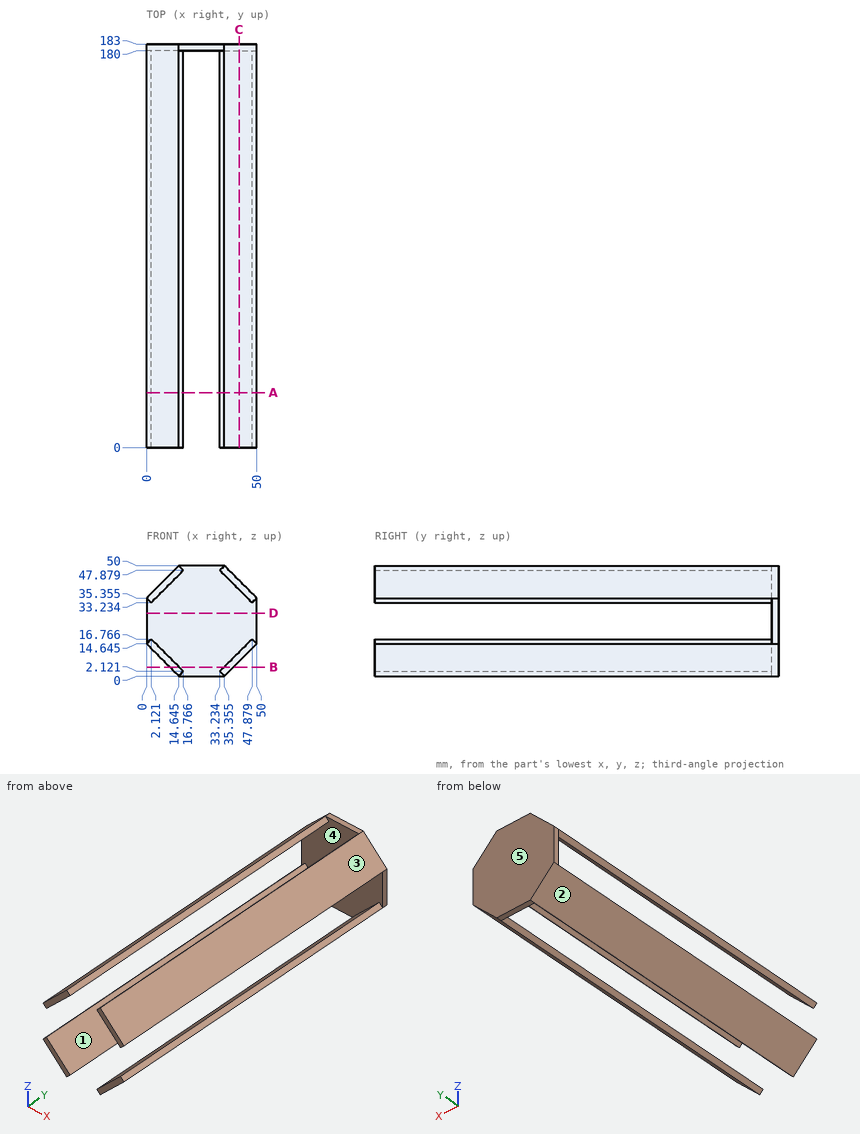
Print and shaded views of the part. All mm, measured from the part's lowest x, y and z. A direction names the side the tool comes from. Coordinates: 2 decimals unless noted, no trailing zeros. Order: outer loops, then holes, each group sorted by start corner. A loop starts at its lowest first (then second) coordinate and runs counter-clockwise, first axis right, second up. Notation, with made-up numbers: (77, -13.5) - (81, -13.5) arc R8 ccw to (81, 1.5) - close; hole circle Ø1 at (51.25, 14). An arc over 180 degrees is marked (long way). Put each result on its own line as item: value.
1. Saw through at D-D (z = 28.5). Write the cut outline in (x, y), and give its area (3 significant figures).
Answer sheet:
outline: (0, 180) - (50, 180) - (50, 183) - (0, 183) - close
area: 150 mm^2
2. Tool access for the marked faces 4 and 5: list every direction of +Z, -Z, +X, -X, +Y, -Y with a clear straight run to the whole face (end or side of a thin tool).
Answer sheet:
face 4: -Y
face 5: +Z, -Z, +X, -X, +Y
3. Drop flat-ended pins along their axis: P1, Ø6, axis at x = 27.5, z = 22.5, coming from the -Y side; P2, Ø1.5, axis at y = 77.5, z = 40, coming from the -X side (1 decimal); P3, Ø10, axis at x = 30, y = 26.5, coming from the -Z side (1 decimal). Give the stop position or say it passes through.
Answer sheet:
P1: stops at y = 180
P2: stops at x = 3.9
P3: stops at z = 0.4
4. Pull direction Z, two halves, no side cores. Call the marked faces 1, 2 and 3: pulls with the +Z half, pulls with the -Z half, needs draft (parallel to the pull), parting line crosses it, or undercut.
Answer sheet:
face 1: undercut
face 2: pulls with the -Z half
face 3: pulls with the +Z half
5. Probe line 1 along Y through (x, z) = (36, 19); line 2 along X through (y, z) = (116, 42.5) (1 decimal); line 3 along Z through (x, y) = (38, 100) (1 decimal). List the from-to ranges inside material, lowest first. Write a range as [from, to].
Answer sheet:
line 1: y = [180, 183]
line 2: x = [7.1, 11.4], [38.6, 42.9]
line 3: z = [2.6, 6.9], [43.1, 47.4]
6. Saw through at C-C (x = 42). Write the cut outline in (y, z) (1 decimal), and give its area (3 significant figures).
Answer sheet:
outline: (0, 6.6) - (183, 6.6) - (183, 43.4) - (0, 43.4) - (0, 39.1) - (180, 39.1) - (180, 10.9) - (0, 10.9) - close
area: 1,640 mm^2
7. Saw through at A-A (y = 25). Write the cut outline in (x, z) (1 decimal).
Answer sheet:
outline: (0, 14.6) - (14.6, 0) - (16.8, 2.1) - (2.1, 16.8) - close; (0, 35.4) - (2.1, 33.2) - (16.8, 47.9) - (14.6, 50) - close; (33.2, 2.1) - (35.4, 0) - (50, 14.6) - (47.9, 16.8) - close; (33.2, 47.9) - (47.9, 33.2) - (50, 35.4) - (35.4, 50) - close
8. Saw through at B-B (z = 4). Write the cut outline in (x, y) (1 decimal).
Answer sheet:
outline: (10.6, 0) - (14.9, 0) - (14.9, 180) - (35.1, 180) - (35.1, 0) - (39.4, 0) - (39.4, 183) - (10.6, 183) - close
